Job drawing, mm, ordinate dimensions from the low corner. One solid piece. Coordinates: 2 decimals unless noted, no trailing zeros. Order: outer loops, then holes, each group sorted by start corner. A loop starts at its lowest first (then second) coordinate and runs counter-clockwise, first axis right, second up. Notation, with made-up numbers: (72.25, -32) - (119.25, -32) arc R24 cw to (119.25, -10) - close; hole circle Ø8 at (49.25, 68). An arc over 180 degrees is marked (long way). Return JSON: item names as keys, results as strings.
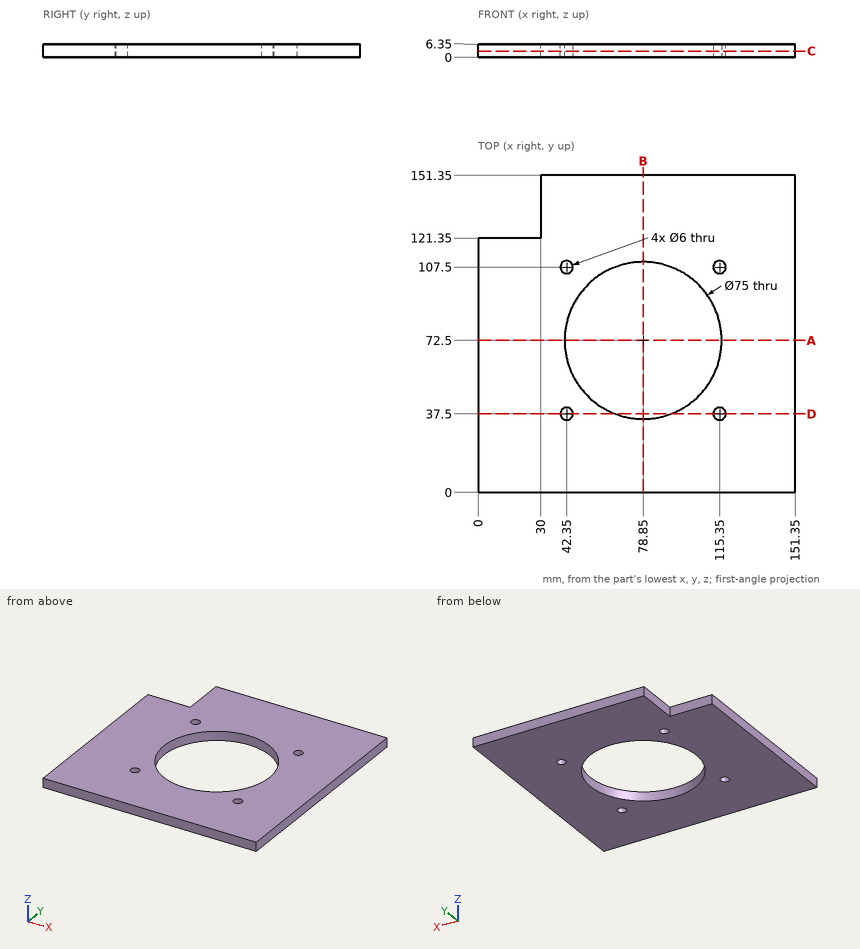
1. Cut at C-C on z = 3. Give the cut face in (x, y).
Check values:
{"outline": "(0, 0) - (151.35, 0) - (151.35, 151.35) - (30, 151.35) - (30, 121.35) - (0, 121.35) - close; hole circle Ø6 at (42.35, 37.5); hole circle Ø6 at (42.35, 107.5); hole circle Ø75 at (78.85, 72.5); hole circle Ø6 at (115.35, 37.5); hole circle Ø6 at (115.35, 107.5)"}
2. Probe L1, parallel to X at y = 105.5, z = 4.5; L2, parallel to Y at x = 89, z = 3; L3, parallel to X at y = 55, z = 2.5. List the from-to ranges inside material, lowest first.
Check values:
{"L1": "0 to 40.11, 44.59 to 61.04, 96.66 to 113.11, 117.59 to 151.35", "L2": "0 to 36.4, 108.6 to 151.35", "L3": "0 to 45.68, 112.02 to 151.35"}
3. Drop flat-ended pins along their axis: pin 1 (8 mm diameter, centred on x = 115.35, y = 107.5, fed in from -Z); pin 2 (1.9 mm diameter, centred on x = 16, z = 2, fed in from +Y). Give the stop position or say it passes through.
Check values:
{"pin 1": "z = 0", "pin 2": "y = 121.35"}
4. Cut at D-D on y = 37.5. Give the cut face in (x, z).
Check values:
{"outline": "(0, 0) - (39.35, 0) - (39.35, 6.35) - (0, 6.35) - close; (45.35, 0) - (65.39, 0) - (65.39, 6.35) - (45.35, 6.35) - close; (92.31, 0) - (112.35, 0) - (112.35, 6.35) - (92.31, 6.35) - close; (118.35, 0) - (151.35, 0) - (151.35, 6.35) - (118.35, 6.35) - close"}
5. Cut at B-B on x = 78.85. Give the cut face in (y, z).
Check values:
{"outline": "(0, 0) - (35, 0) - (35, 6.35) - (0, 6.35) - close; (110, 0) - (151.35, 0) - (151.35, 6.35) - (110, 6.35) - close"}
6. Cut at A-A on y = 72.5. Give the cut face in (x, z), plus the area to 3 significant figures.
Check values:
{"outline": "(0, 0) - (41.35, 0) - (41.35, 6.35) - (0, 6.35) - close; (116.35, 0) - (151.35, 0) - (151.35, 6.35) - (116.35, 6.35) - close", "area": "485 mm²"}
